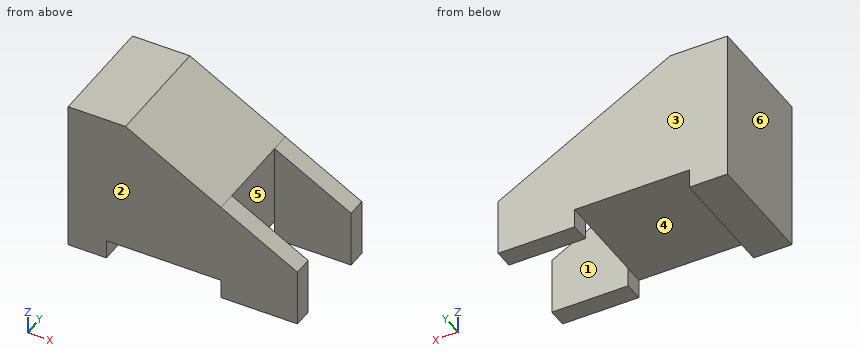
```python
from build123d import *

# Parameters (mm, degrees)
F1_DEPTH = 7.5
F2_W     = 15
F2_H     = 2.5
F3_DEPTH = 15.001
F4_DEPTH = 5


with BuildPart() as f1:
    # F0 (on Front) → F1 (new body, symmetric)
    with BuildSketch(Plane.XZ):
        Polygon((0, 20), (0, 0), (20, 0), (20, 13.0555555556), (7.5, 20), align=None)
        Polygon((20, 13.0555555556), (20, 0), (30, 0), (30, 7.5), align=None)
    extrude(amount=F1_DEPTH, both=True)

    # F2 (on face) → F3 (cut, through all)
    with BuildSketch(Plane.XZ.offset(7.5)):
        with Locations((12.5, 1.25)):
            Rectangle(F2_W, F2_H)
    extrude(amount=-F3_DEPTH, mode=Mode.SUBTRACT)

    # F0 (on Front) → F4 (cut, symmetric)
    with BuildSketch(Plane.XZ):
        Polygon((20, 13.0555555556), (20, 0), (30, 0), (30, 7.5), align=None)
    extrude(amount=F4_DEPTH, both=True, mode=Mode.SUBTRACT)


solid = f1.part
```
For this review, take the finished solid that the model builds, in its own axes (mm). Face numbers are marked on the shaded views. A direction names the side the tool comes from. Round coordinates to 2 decimals unless told otherwise and drop trailing zeros. Write each loop counter-clockwise with the first axis right and the second up, starting at its lowest first coordinate (ties: lowest second). Pieces come first, ordered by that corner, then holes.
1) Take a section at B-B on z = 5.5. Give the boundary of the cut face in (x, y).
Answer below:
outline: (0, -7.5) - (30, -7.5) - (30, -5) - (20, -5) - (20, 5) - (30, 5) - (30, 7.5) - (0, 7.5) - close
2) Mouldability with a two-part tool opening along Y and no side actions: class the marked faces 1, 2 and 3 as +Y half, -Y half, draft (parallel to the pull), parting line (faces both ways), or undercut.
Answer below:
face 1: undercut
face 2: -Y half
face 3: +Y half
3) Take a section at D-D on z = 12.5. Give the boundary of the cut face in (x, y).
Answer below:
outline: (0, -7.5) - (21, -7.5) - (21, -5) - (20, -5) - (20, 5) - (21, 5) - (21, 7.5) - (0, 7.5) - close
4) Machinability: for the marked faces 4, 5 and 6, which of the approach directions +Z, -Z, +X, -X, +Y, -Y give a long, thin tool a straight path to every point of the face, cutting with its end or side? Answer none if there is none.
Answer below:
face 4: -Z, +Y, -Y
face 5: +Z, -Z, +X
face 6: +Z, -Z, -X, +Y, -Y
5) Insertion check: pin 1 Ø1 at (x, y) = (7.5, 2.5) entering from -Z; pin 2 Ø3 at (y, z) = (-7, 1.5) entering from -X. Each pin has a flat end and moves straight along its axis. Give the tip position at first contact, or say it passes through.
Answer below:
pin 1: stops at z = 2.5
pin 2: stops at x = 0
6) For line 1 along Z through (x, y) = (5.25, -6.25); line 2 along X through (y, z) = (-4.5, 12.75); line 3 along X through (y, z) = (-1, 2.25), list the stretches that pass through material, from the lowest coordinate up.
Answer below:
line 1: z = 2.5 to 20
line 2: x = 0 to 20
line 3: x = 0 to 5
7) Take a section at A-A on y = -5.5. Give the boundary of the cut face in (x, z), then the cut area to 3 significant figures.
Answer below:
outline: (0, 0) - (5, 0) - (5, 2.5) - (20, 2.5) - (20, 0) - (30, 0) - (30, 7.5) - (7.5, 20) - (0, 20) - close
area: 422 mm2
8) Take a section at C-C on x = 22.5. Give the boundary of the cut face in (y, z), then the cut area to 3 significant figures.
Answer below:
outline: (-7.5, 0) - (-5, 0) - (-5, 11.67) - (-7.5, 11.67) - close; (5, 0) - (7.5, 0) - (7.5, 11.67) - (5, 11.67) - close
area: 58.3 mm2
